The model under review builds one solid part; all positions refer to its coordinate system, in mm. Face numbers are marked on the shaded views. Give positions to 0.01 mm unless a question says otherwise; leave off trailing zeros. Order: outer loops, then holes, each group sorted by start corner. A loop starts at its lowest first (then second) coordinate and runs counter-clockwise, first axis right, second up.
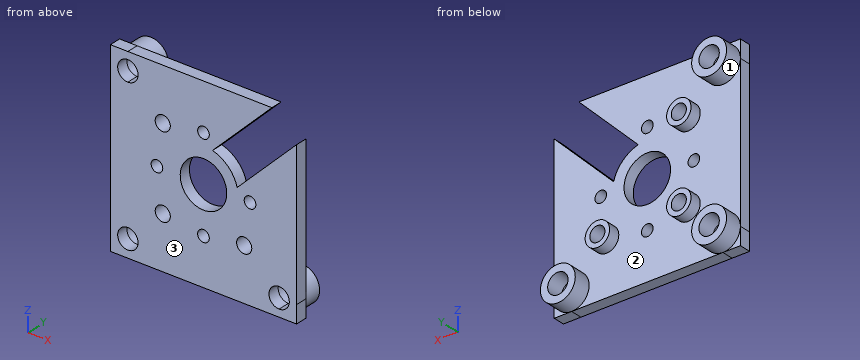
```python
from build123d import *

# Parameters (mm, degrees)
SKETCH_1_W          = 32
SKETCH_1_H          = 32
SKETCH_1_R          = 1
SKETCH_1_R_2        = 4
SKETCH_1_R_3        = 1.75
EXTRUDE_1_DEPTH     = 2
SKETCH_2_R          = 2.1
SKETCH_2_R_2        = 1.3
EXTRUDE_3_DEPTH     = 2
CUT_EXTRUDE_START   = -2
SKETCH_2_6_R        = 1.3
SKETCH_2_6_R_2      = 1.75
SKETCH_2_6_R_3      = 2.1
CUT_EXTRUDE_2_DEPTH = 2
SKETCH_3_R          = 3
SKETCH_3_R_2        = 1.75
EXTRUDE_5_DEPTH     = 5


with BuildPart() as part:
    # 草图1 → 凸台-拉伸1 (new body)
    with BuildSketch(Plane(origin=(0, 0, 0), x_dir=(1, 0, 0), z_dir=(0, 1, 0))):
        Rectangle(SKETCH_1_W, SKETCH_1_H)
        with Locations(Location((8, 0, 0), (0, 0, 270))):
            Circle(SKETCH_1_R, mode=Mode.SUBTRACT)
        with Locations(Location((0, -8, 0), (0, 0, 270))):
            Circle(SKETCH_1_R, mode=Mode.SUBTRACT)
        with Locations(Location((-8, 0, 0), (0, 0, 270))):
            Circle(SKETCH_1_R, mode=Mode.SUBTRACT)
        with Locations(Location((0, 8, 0), (0, 0, 270))):
            Circle(SKETCH_1_R, mode=Mode.SUBTRACT)
        with Locations(Location((0, 0, 0), (0, 0, 270))):
            Circle(SKETCH_1_R_2, mode=Mode.SUBTRACT)
        with Locations(Location((13, 13, 0), (0, 0, 270))):
            Circle(SKETCH_1_R_3, mode=Mode.SUBTRACT)
        with Locations(Location((-13, 13, 0), (0, 0, 270))):
            Circle(SKETCH_1_R_3, mode=Mode.SUBTRACT)
        with Locations(Location((13, -13, 0), (0, 0, 270))):
            Circle(SKETCH_1_R_3, mode=Mode.SUBTRACT)
        with Locations(Location((-13, -13, 0), (0, 0, 270))):
            Circle(SKETCH_1_R_3, mode=Mode.SUBTRACT)
    extrude(amount=EXTRUDE_1_DEPTH)

    # 草图2 → 凸台-拉伸3 (add)
    # profile 1 of 3: a face of its own
    with BuildSketch(Plane(origin=(0, 2, 0), x_dir=(1, 0, 0), z_dir=(0, 1, 0))):
        with Locations(Location((-7, -7, 0), (0, 0, 270))):
            Circle(SKETCH_2_R)
        with Locations(Location((-7, -7, 0), (0, 0, 270))):
            Circle(SKETCH_2_R_2, mode=Mode.SUBTRACT)
    # profile 2 of 3: a face of its own
    with BuildSketch(Plane(origin=(0, 2, 0), x_dir=(1, 0, 0), z_dir=(0, 1, 0))):
        with Locations(Location((-7, 7, 0), (0, 0, 270))):
            Circle(SKETCH_2_R)
        with Locations(Location((-7, 7, 0), (0, 0, 270))):
            Circle(SKETCH_2_R_2, mode=Mode.SUBTRACT)
    # profile 3 of 3: a face of its own
    with BuildSketch(Plane(origin=(0, 2, 0), x_dir=(1, 0, 0), z_dir=(0, 1, 0))):
        with Locations(Location((7, 7, 0), (0, 0, 270))):
            Circle(SKETCH_2_R)
        with Locations(Location((7, 7, 0), (0, 0, 270))):
            Circle(SKETCH_2_R_2, mode=Mode.SUBTRACT)
    extrude(amount=EXTRUDE_3_DEPTH)

    # 草图2<6> → 切除-拉伸2 (cut)
    # profile 1 of 6: a face of its own
    with BuildSketch(Plane(origin=(0, 2, 0), x_dir=(1, 0, 0), z_dir=(0, 1, 0)).offset(CUT_EXTRUDE_START)):
        with Locations(Location((-7, 7, 0), (0, 0, 270))):
            Circle(SKETCH_2_6_R)
    # profile 2 of 6: a face of its own
    with BuildSketch(Plane(origin=(0, 2, 0), x_dir=(1, 0, 0), z_dir=(0, 1, 0)).offset(CUT_EXTRUDE_START)):
        with Locations(Location((-7, -7, 0), (0, 0, 270))):
            Circle(SKETCH_2_6_R)
    # profile 3 of 6: a face of its own
    with BuildSketch(Plane(origin=(0, 2, 0), x_dir=(1, 0, 0), z_dir=(0, 1, 0)).offset(CUT_EXTRUDE_START)):
        with Locations(Location((7, 7, 0), (0, 0, 270))):
            Circle(SKETCH_2_6_R)
    # profile 4 of 6: a face of its own
    with BuildSketch(Plane(origin=(0, 2, 0), x_dir=(1, 0, 0), z_dir=(0, 1, 0)).offset(CUT_EXTRUDE_START)):
        with BuildLine():
            Line((16, -11.757359313), (5.795554958, -1.552914271))
            ThreePointArc((5.795554958, -1.552914271), (4.242640687, -4.242640687), (1.552914271, -5.795554958))
            Line((1.552914271, -5.795554958), (11.757359313, -16))
            Line((11.757359313, -16), (16, -16))
            Line((16, -16), (16, -11.757359313))
        make_face()
        with Locations((13, -13)):
            Circle(SKETCH_2_6_R_2, mode=Mode.SUBTRACT)
        with Locations((7, -7)):
            Circle(SKETCH_2_6_R_3, mode=Mode.SUBTRACT)
    # profile 5 of 6: a face of its own
    with BuildSketch(Plane(origin=(0, 2, 0), x_dir=(1, 0, 0), z_dir=(0, 1, 0)).offset(CUT_EXTRUDE_START)):
        with Locations((7, -7)):
            Circle(SKETCH_2_6_R_3)
        with Locations((7, -7)):
            Circle(SKETCH_2_6_R, mode=Mode.SUBTRACT)
    # profile 6 of 6: a face of its own
    with BuildSketch(Plane(origin=(0, 2, 0), x_dir=(1, 0, 0), z_dir=(0, 1, 0)).offset(CUT_EXTRUDE_START)):
        with Locations((7, -7)):
            Circle(SKETCH_2_6_R)
    extrude(amount=CUT_EXTRUDE_2_DEPTH, mode=Mode.SUBTRACT)

    # 草图3 → 凸台-拉伸5 (add)
    # profile 1 of 3: a face of its own
    with BuildSketch(Plane.XZ):
        with Locations(Location((-13, 13, 0), (0, 0, 270))):
            Circle(SKETCH_3_R)
        with Locations(Location((-13, 13, 0), (0, 0, 270))):
            Circle(SKETCH_3_R_2, mode=Mode.SUBTRACT)
    # profile 2 of 3: a face of its own
    with BuildSketch(Plane.XZ):
        with Locations(Location((-13, -13, 0), (0, 0, 270))):
            Circle(SKETCH_3_R)
        with Locations(Location((-13, -13, 0), (0, 0, 90))):
            Circle(SKETCH_3_R_2, mode=Mode.SUBTRACT)
    # profile 3 of 3: a face of its own
    with BuildSketch(Plane.XZ):
        with Locations(Location((13, -13, 0), (0, 0, 270))):
            Circle(SKETCH_3_R)
        with Locations(Location((13, -13, 0), (0, 0, 270))):
            Circle(SKETCH_3_R_2, mode=Mode.SUBTRACT)
    extrude(amount=-EXTRUDE_5_DEPTH)


solid = part.part
```
Item 1: For line 1 (Z direction, x = -13, y = 4.45); line 2 (X direction, y = 1.3, z = 0), list the stretches that pass through material, from the lowest coordinate up.
Values found:
line 1: z = -16 to -14.75, -11.25 to -10, 10 to 11.25, 14.75 to 16
line 2: x = -16 to -9, -7 to -4, 4 to 7, 9 to 16
Item 2: Draft analysis for pull direction X (two halves, no side actions). For the marked faces 1, 2 and 3, state which applies: released by +X, released by -X, zero draft, split by the parting line, or undercut.
Values found:
face 1: split by the parting line
face 2: undercut
face 3: zero draft
Item 3: Clearance check with flat-ended pins moving along their axes: pin 1 Ø4.5 at (x, z) = (8, -7.5) entering from +Y; pin 2 Ø1.5 at (x, z) = (-4, 8.5) entering from -Y; pin 3 Ø3 at (x, z) = (-8, 0) entering from +Y. State where each tip first meets the part, or that it passes through.
Values found:
pin 1: stops at y = 4
pin 2: stops at y = 0
pin 3: stops at y = 2
Item 4: Take a section at B-B (x = 12.5). Give the boundary of the cut face in (y, z).
Values found:
outline: (0, -16) - (2, -16) - (2, -15.96) - (5, -15.96) - (5, -14.68) - (0, -14.68) - close; (0, -11.32) - (5, -11.32) - (5, -10.04) - (2, -10.04) - (2, 8.26) - (0, 8.26) - close
Item 5: Take a section at A-A (z = 0). Give the boundary of the cut face in (x, y), and give its area (3 significant figures).
Values found:
outline: (-16, 0) - (-9, 0) - (-9, 2) - (-16, 2) - close; (-7, 0) - (-4, 0) - (-4, 2) - (-7, 2) - close; (4, 0) - (7, 0) - (7, 2) - (4, 2) - close; (9, 0) - (16, 0) - (16, 2) - (9, 2) - close
area: 40.0 mm2
